from build123d import *

# Parameters (mm, degrees)
F0_W     = 79.502
F0_H     = 117.602
F1_DEPTH = 12.7
F2_R     = 1.778
F3_DEPTH = 12.701
F4_R     = 21.209
F5_DEPTH = 36.322
F6_R     = 21.209
F7_DEPTH = 24.638


with BuildPart() as f1:
    # F0 (on Front) → F1 (new body)
    with BuildSketch(Plane.XZ):
        Rectangle(F0_W, F0_H)
    extrude(amount=F1_DEPTH)

    # F2 (on face) → F3 (cut, through all)
    with BuildSketch(Plane.XZ.offset(12.7)):
        with Locations((-23.749, 41.275)):
            Circle(F2_R)
        with Locations((23.749, 41.275)):
            Circle(F2_R)
        with Locations((-23.749, -41.275)):
            Circle(F2_R)
        with Locations((23.749, -41.275)):
            Circle(F2_R)
    extrude(amount=-F3_DEPTH, mode=Mode.SUBTRACT)

    # F4 (on face) → F5 (join)
    with BuildSketch(Plane(origin=(0, 0, 0), x_dir=(-1, 0, 0), z_dir=(0, 1, 0))):
        with Locations((0, 25.908)):
            Circle(F4_R)
        with Locations((0, -25.908)):
            Circle(F4_R)
    extrude(amount=F5_DEPTH)

    # F6 (on face) → F7 (join)
    with BuildSketch(Plane.XZ.offset(12.7)):
        with Locations((0, 25.908)):
            Circle(F6_R)
        with Locations((0, -25.908)):
            Circle(F6_R)
    extrude(amount=F7_DEPTH)


solid = f1.part
Read the model definition and answer for the solid it produces. Units are mm, in the model's axes. A direction names the side the tool comes from. Round coordinates to 2 decimals unless told otherwise and drop trailing zeros. Loops run counter-clockwise (first coordinate to the right, second up) from the corner with the lowest first, then second, coordinate; pieces in that order, holes last. Notation, with made-up numbers: (62.5, 61) - (111.5, 61) arc R38 cw to (111.5, 100) - close; hole circle Ø6 at (2, 43.5). An arc over 180 degrees is marked (long way). One line per question, with ' | ' between items. Start each with the question number.
Q1. Section B-B on y = -25 is taken. Give the vertices of the cut face in (x, z), plus the area to 3 significant figures.
Q2. Section D-D on x = -31 is taken. Give the vertices of the cut face in (y, z), plus the area to 3 significant figures.
Q3. For a pull along X with two mould halves and no side action, classify faces 1 (the flat face through (0, -37.338, 26)), 2 (the cylindrical face through (-20.23, 17.91, 32.28)), 3 (the flat face through (-39.751, -6, -1)), 4 (the cylindrical face through (23.52, -6.44, 43.04)) as +X half, -X half, draft (parallel to the pull), parting line (faces both ways), or undercut.
Q4. Section C-C on z = -13.5 is taken. Give the vertices of the cut face in (x, y), plus the area to 3 significant figures.
Q5. Section A-A on x = 0 is taken. Give the vertices of the cut face in (y, z).
Q6. For faces 5 (the cylindrical face through (4.598, 17.907, -46.613)), 6 (the cylindrical face through (20.23, -24.85, 32.28)), 7 (the flat face through (39.751, -6, -1)), determine the directions among +Z, -Z, +X, -X, +Y, -Y from which every point of the face is accessible in a straight line to the end or side of a thin tool.
Q7. Find the intervals of material crossed by L1, parallel to Y at x = -35, z = -47; L2, parallel to Z at x = 0, y = -25; L3, parallel to Z at x = -3, y = 30, in increasing order.
Q8. Flat-ended cylindrical pins translate along their axes: pin 1 (4 mm diameter, centred on x = 23.749, z = 41.275, fed in from -Y); pin 2 (4 mm diameter, centred on x = 23.749, z = -41.275, fed in from +Y); pin 3 (1.5 mm diameter, centred on x = 13, y = -18.5, fed in from +Z). Find the tip coordinate at first contact, or state that the pin passes through.
Established:
1) outline: circle Ø42.42 at (0, -25.91); circle Ø42.42 at (0, 25.91) | area: 2,830 mm²
2) outline: (-12.7, -58.8) - (0, -58.8) - (0, 58.8) - (-12.7, 58.8) - close | area: 1,490 mm²
3) face 1: draft | face 2: parting line | face 3: -X half | face 4: undercut
4) outline: (-39.75, -12.7) - (-17.2, -12.7) - (-17.2, -37.34) - (17.2, -37.34) - (17.2, -12.7) - (39.75, -12.7) - (39.75, 0) - (17.2, 0) - (17.2, 36.32) - (-17.2, 36.32) - (-17.2, 0) - (-39.75, 0) - close | area: 3,110 mm²
5) outline: (-37.34, -47.12) - (-12.7, -47.12) - (-12.7, -58.8) - (0, -58.8) - (0, -47.12) - (36.32, -47.12) - (36.32, -4.7) - (0, -4.7) - (0, 4.7) - (36.32, 4.7) - (36.32, 47.12) - (0, 47.12) - (0, 58.8) - (-12.7, 58.8) - (-12.7, 47.12) - (-37.34, 47.12) - (-37.34, 4.7) - (-12.7, 4.7) - (-12.7, -4.7) - (-37.34, -4.7) - close
6) face 5: +Y | face 6: -Y | face 7: +Z, -Z, +X, +Y, -Y
7) L1: -12.7 to 0 | L2: -47.12 to -4.7, 4.7 to 47.12 | L3: -46.9 to -4.91, 4.91 to 46.9
8) pin 1: y = -12.7 | pin 2: y = 0 | pin 3: z = 43.22
